Part print with two shaded views. Sizes in mm from the minimum x, y, z corner. A direction names the side the tool comes from. Give positions to 0.01 mm unless a question says otherwise; leave off trailing zeros. Order: outer loops, then holes, each group sorted by start corner. A loop starts at its lowest first (then second) coordinate and runs counter-clockwise, first axis right, second up. Notation, with made-up numbers: (-23.5, 8.25) -> (27.5, 8.25) arc R13 ccw to (27.5, 29.25) -> close; hole circle Ø4 at (-29.75, -26). An arc over 180 degrees is marked (long way). Answer as CSV lines item,"result".
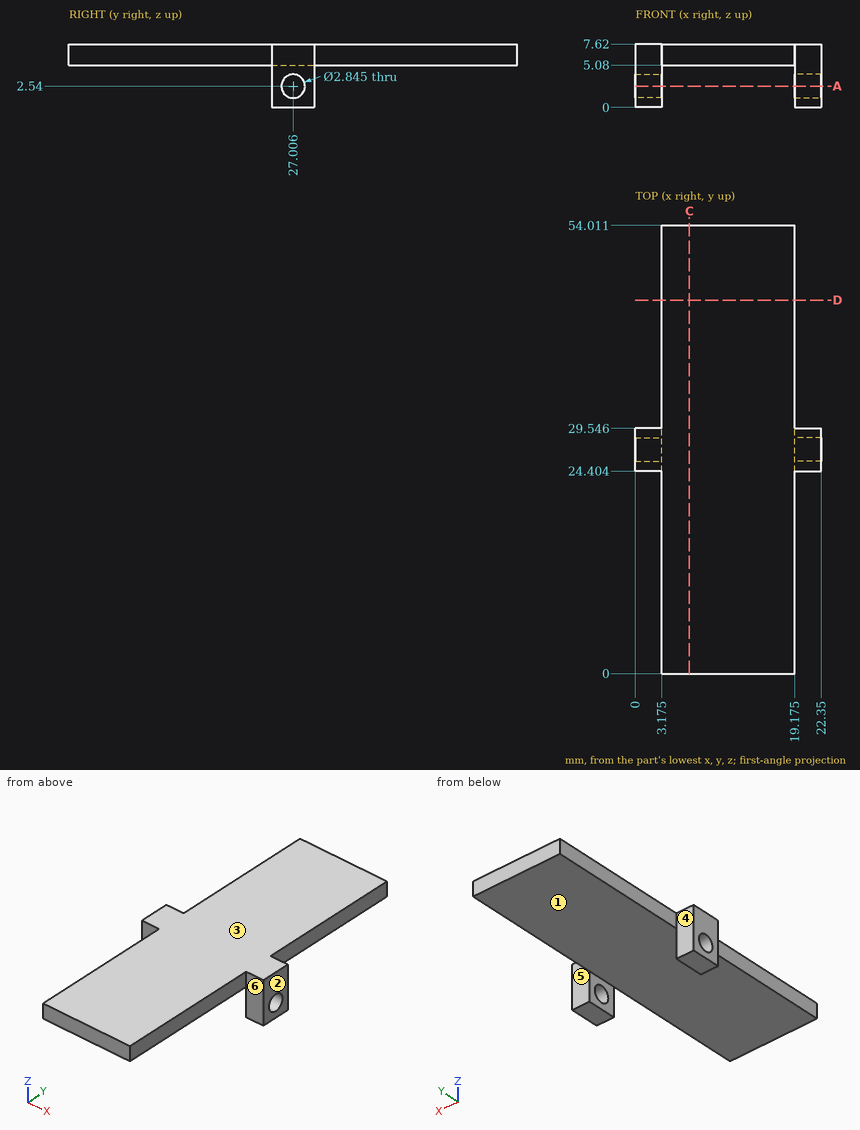
1) Pin check, flat tips, straight feed: P1, Ø3.5, axis at x = 21, z = 3.5, coming from the -Y side; P2, Ø1.3, axis at y = 40, z = 6.5, coming from the +X side (3 decimals); P3, Ø0.8, axis at y = 15, z = 6, coming from the -X side (3 decimals). Stop position of each tip, or through.
Data:
P1,"stops at y = 24.4"
P2,"stops at x = 19.175"
P3,"stops at x = 3.175"
2) Band-saw the part on A-A, the plane z = 2.54. Give the number of separate pieces and of enclosed holes in the cut face, then the cut area to 3 significant figures.
Data:
separate pieces,"4"
enclosed holes,"0"
area,"14.6 mm2"
3) Band-saw the part on C-C, the plane x = 6.5. Write the cut outline in (y, z).
Data:
outline,"(0, 5.08) -> (54.01, 5.08) -> (54.01, 7.62) -> (0, 7.62) -> close"
4) Pull direction Z, two halves, no side cores. Call the marked faces 1, 2 and 3: pulls with the +Z half, pulls with the -Z half, needs draft (parallel to the pull), parting line crosses it, or undercut.
Data:
face 1,"pulls with the -Z half"
face 2,"needs draft"
face 3,"pulls with the +Z half"
5) Wall check: line 1 along Y through (x, z) = (0.8, 2.54) (1 decimal); line 2 along Y through (x, z) = (21.5, 7.25) (1 decimal); line 3 along Z through (x, y) = (10.5, 24.5). Give the ranges that are in metal, low to high. Write a range as [from, to].
Data:
line 1,"y = [24.4, 25.6], [28.4, 29.5]"
line 2,"y = [24.4, 29.5]"
line 3,"z = [5.08, 7.62]"
6) Band-saw the part on D-D, the plane y = 45. Write the cut outline in (x, z) (1 decimal).
Data:
outline,"(3.2, 5.1) -> (19.2, 5.1) -> (19.2, 7.6) -> (3.2, 7.6) -> close"
7) Which spindle directions (+Z, -Z, +X, -X, +Y, -Y) get a long thin tool onto all of the face, cutting with end or side? Do the marked faces 4, 5 and 6. Say none if no direction does.
Data:
face 4,"+Z, -Z, -X, +Y"
face 5,"+Z, -Z, +X, +Y"
face 6,"+Z, -Z, +X, -Y"
